from build123d import *

# Parameters (mm, degrees)
SKETCH_1_R               = 4
EXTRUDE_1_DEPTH          = 16
SKETCH_2_R               = 1.95
CUT_EXTRUDE_1_DEPTH      = 17.970562748
PATTERN_CIRCULAR_1_COUNT = 4
SKETCH_3_W               = 4.5
SKETCH_3_H               = 4.5
EXTRUDE_3_DEPTH          = 16
EXTRUDE_START            = 1
SKETCH_5_R               = 4
EXTRUDE_5_DEPTH          = 1
SKETCH_6_R               = 17.5
EXTRUDE_6_DEPTH          = 3
SKETCH_7_R               = 7.5
CUT_EXTRUDE_2_DEPTH      = 1.8
FILLET_1_R               = 1
SKETCH_8_R               = 1.3
CUT_EXTRUDE_3_DEPTH      = 31.024989649
SKETCH_9_R               = 2.5
SKETCH_9_R_2             = 1.3
CUT_EXTRUDE_4_DEPTH      = 1
PATTERN_CIRCULAR_2_COUNT = 8


with BuildPart() as part:
    # Sketch 1 → Extrude 1 (new body)
    with BuildSketch(Plane(origin=(0, 0, 0), x_dir=(1, 0, 0), z_dir=(0, 1, 0))):
        with Locations(Location((0, 0, 0), (0, 0, 270))):
            Circle(SKETCH_1_R)
    extrude(amount=EXTRUDE_1_DEPTH)

    # Sketch 2 → Cut-Extrude 1 (cut, symmetric)
    with BuildSketch(Plane.XY):
        with Locations(Location((0, 12, 0), (0, 0, 90.000000018))):
            Circle(SKETCH_2_R)
        with Locations(Location((0, 4, 0), (0, 0, 90.000000018))):
            Circle(SKETCH_2_R)
    cut_extrude_1 = extrude(amount=CUT_EXTRUDE_1_DEPTH, both=True, mode=Mode.SUBTRACT)

    # Pattern Circular 1: Cut-Extrude 1 ×4 about axis
    pattern_circular_1_axis = Axis((0, 16, 0), (0, 1, 0))
    for i in range(1, PATTERN_CIRCULAR_1_COUNT):
        add(cut_extrude_1.rotate(pattern_circular_1_axis, i * 360 / PATTERN_CIRCULAR_1_COUNT), mode=Mode.SUBTRACT)



with BuildPart() as body_2:
    # Sketch 3 → Extrude 3 (new body)
    with BuildSketch(Plane(origin=(0, 16, 0), x_dir=(1, 0, 0), z_dir=(0, 1, 0))):
        Rectangle(SKETCH_3_W, SKETCH_3_H)
    extrude(amount=-EXTRUDE_3_DEPTH)


with BuildPart() as part_1:
    add(part.part)

    add(body_2.part)  # Extrude 5 merges body 2
    # Sketch 5 → Extrude 5 (add)
    with BuildSketch(Plane.XZ.offset(EXTRUDE_START)):
        with Locations(Location((0, 0, 0), (0, 0, 270))):
            Circle(SKETCH_5_R)
    extrude(amount=-EXTRUDE_5_DEPTH)

    # Sketch 6 → Extrude 6 (add)
    with BuildSketch(Plane.XZ.offset(1)):
        with Locations(Location((0, 0, 0), (0, 0, 270))):
            Circle(SKETCH_6_R)
    extrude(amount=EXTRUDE_6_DEPTH)

    # Sketch 7 → Cut-Extrude 2 (cut)
    with BuildSketch(Plane.XZ.offset(4)):
        with Locations(Location((0, 0, 0), (0, 0, 270))):
            Circle(SKETCH_7_R)
    extrude(amount=-CUT_EXTRUDE_2_DEPTH, mode=Mode.SUBTRACT)

    # Fillet 1
    fillet_1_edges = [part_1.edges().sort_by_distance(p)[0] for p in [
        (0, -1, 4),
    ]]
    fillet(fillet_1_edges, radius=FILLET_1_R - 0.0001)  # a hair under: the kernel refuses the full size

    # Sketch 8 → Cut-Extrude 3 (cut, through all)
    with BuildSketch(Plane(origin=(0, -1, 0), x_dir=(1, 0, 0), z_dir=(0, 1, 0))):
        with Locations(Location((-12, 0, 0), (0, 0, 270))):
            Circle(SKETCH_8_R)
    cut_extrude_3 = extrude(amount=-CUT_EXTRUDE_3_DEPTH, mode=Mode.SUBTRACT)

    # Sketch 9 → Cut-Extrude 4 (cut)
    with BuildSketch(Plane(origin=(0, -1, 0), x_dir=(1, 0, 0), z_dir=(0, 1, 0))):
        with Locations(Location((-12, 0, 0), (0, 0, 270))):
            Circle(SKETCH_9_R)
        with Locations(Location((-12, 0, 0), (0, 0, 270))):
            Circle(SKETCH_9_R_2, mode=Mode.SUBTRACT)
    cut_extrude_4 = extrude(amount=-CUT_EXTRUDE_4_DEPTH, mode=Mode.SUBTRACT)

    # Pattern Circular 2: Cut-Extrude 3, Cut-Extrude 4 ×8 about axis
    pattern_circular_2_axis = Axis((0, 0, 0), (0, 1, 0))
    add([cut_extrude_3.rotate(pattern_circular_2_axis, i * 360 / PATTERN_CIRCULAR_2_COUNT) for i in range(1, PATTERN_CIRCULAR_2_COUNT)], mode=Mode.SUBTRACT)
    add([cut_extrude_4.rotate(pattern_circular_2_axis, i * 360 / PATTERN_CIRCULAR_2_COUNT) for i in range(1, PATTERN_CIRCULAR_2_COUNT)], mode=Mode.SUBTRACT)


solid = part_1.part
Verification items for the finished model (mm, model axes). A direction names the side the tool comes from. Coordinates: 2 decimals unless noted, no trailing zeros. Order: outer loops, then holes, each group sorted by start corner. A loop starts at its lowest first (then second) coordinate and runs counter-clockwise, first axis right, second up. Notation, with made-up numbers: M 62,36.25 L 74,36.25 A34 cw 74,66.25 Z; hole C 61.5,37.5 d2. An arc over 180 degrees is marked long. One line per item, written item: value. Start each with the question number.
Item 1: Sectioned sample at D-D on z = 0. Give the number of separate pieces and of enclosed holes in the cut face, then the cut area to 3 significant figures.
Item 2: Thickness scan on probe 1 along X at (y, z) = (-3.45, 0); probe 2 along Y at (x, z) = (0, -2.9); probe 3 along Y at (x, z) = (3.5, 1). Record the ranges inside material, lowest first.
Item 3: Sectioned sample at B-B on y = 5.25. Record the cut outline in (x, z), then the cut area to 3 significant figures.
Item 4: Depth check by flat-ended pin: P1, Ø2, axis at x = 1, y = 3.5, coming from the -Z side; P2, Ø1.6, axis at x = -8.49, z = -8.49, coming from the +Y side; P3, Ø1.5, axis at x = -12.5, y = -0.5, coming from the +Z side; P4, Ø3, axis at y = 6.5, z = 1, coming from the +X side. Enter the tip coordinate at first touch or a pass-through.
Item 5: Mould release check, pull along X, two halves, no side actions. Record for faces 6 (the flat face through (-1.1, -2, -13.1)), 7 (the flat face through (0, 16, 0)), 8 (the flat face through (2.25, 12, 0)), 9 (the cylindrical face through (-10.648, -2.479, 13.887)): pulls with the +X half, pulls with the -X half, needs draft (parallel to the pull), parting line crosses it, or undercut.
Item 6: Sectioned sample at C-C on x = -8.5. Record the cut outline in (y, z), then the cut area to 3 significant figures.
Item 7: Sectioned sample at A-A on z = 12. Record the cut outline in (x, y).
Item 8: Access from +Z, -Z, +X, -X, +Y, -Y to the whole of each face (thin tool, end or side, straight path). Record for faces 1 (the flat face through (13.1, -2, -1.1)), 2 (the flat face through (0, 4, -2.25)), 3 (the cylindrical face through (-2.92, 13.86, 0.59)), 4 (the flat face through (2.25, 4, 0)), 5 (the cylindrical face through (0.75, 13.8, 2.92)).
Calculated:
1. separate pieces: 3
1. enclosed holes: 0
1. area: 167 mm^2
2. probe 1: -17.5 to -13.3, -10.7 to -7.5, 7.5 to 10.7, 13.3 to 17.5
2. probe 2: -2.2 to 2.05, 5.95 to 10.05, 13.95 to 16
2. probe 3: -2.2 to 2.33, 5.67 to 10.33, 13.67 to 16
3. outline: M -3.71,-1.5 A4 ccw -1.5,-3.71 L -1.5,-2.25 L 1.5,-2.25 L 1.5,-3.71 A4 ccw 3.71,-1.5 L 2.25,-1.5 L 2.25,1.5 L 3.71,1.5 A4 ccw 1.5,3.71 L 1.5,2.25 L -1.5,2.25 L -1.5,3.71 A4 ccw -3.71,1.5 L -2.25,1.5 L -2.25,-1.5 Z
3. area: 30.5 mm^2
4. P1: z = -3.78
4. P2: through
4. P3: z = 12.79
4. P4: x = 4
5. face 6: undercut
5. face 7: needs draft
5. face 8: pulls with the +X half
5. face 9: parting line crosses it
6. outline: M -4,-15.3 L -1,-15.3 L -1,-10.99 L -2,-10.99 L -2,-9.79 L -4,-9.79 Z; M -4,-7.19 L -2,-7.19 L -2,-5.99 L -1,-5.99 L -1,5.99 L -2,5.99 L -2,7.19 L -4,7.19 Z; M -4,9.79 L -2,9.79 L -2,10.99 L -1,10.99 L -1,15.3 L -4,15.3 Z
6. area: 71.4 mm^2
7. outline: M -12.74,-4 L -1.3,-4 L -1.3,-2 L -2.5,-2 L -2.5,-1 L -12.74,-1 Z; M 1.3,-4 L 12.74,-4 L 12.74,-1 L 2.5,-1 L 2.5,-2 L 1.3,-2 Z
8. face 1: +Y
8. face 2: -Z
8. face 3: -X
8. face 4: +X
8. face 5: +Z
